from build123d import *

# Parameters (mm, degrees)
SKETCH1_R           = 78.35
SKETCH1_R_2         = 4
SKETCH1_R_3         = 3
SKETCH1_R_4         = 2.5
SKETCH1_W           = 100
SKETCH1_H           = 100
BOSS_EXTRUDE1_DEPTH = 3


with BuildPart() as part:
    # Sketch1 → Boss-Extrude1 (new body)
    with BuildSketch(Plane(origin=(0, 0, 0), x_dir=(1, 0, 0), z_dir=(0, 1, 0))):
        with Locations(Location((0, 0, 0), (0, 0, 270))):
            Circle(SKETCH1_R)
        with Locations(Location((-62.5, 0, 0), (0, 0, 270))):
            Circle(SKETCH1_R_2, mode=Mode.SUBTRACT)
        with Locations(Location((0, -62.5, 0), (0, 0, 270))):
            Circle(SKETCH1_R_3, mode=Mode.SUBTRACT)
        with Locations(Location((0, 62.5, 0), (0, 0, 270))):
            Circle(SKETCH1_R_4, mode=Mode.SUBTRACT)
        with Locations(Location((62.5, 0, 0), (0, 0, 270))):
            Circle(SKETCH1_R_2, mode=Mode.SUBTRACT)
        Rectangle(SKETCH1_W, SKETCH1_H, mode=Mode.SUBTRACT)
    extrude(amount=BOSS_EXTRUDE1_DEPTH)


solid = part.part
Check sheet for the modelled part. Datum: model origin and axes. Units: mm. Give positions to 0.01 mm unless a question says otherwise; leave off trailing zeros. Loops run counter-clockwise (first coordinate to the right, second up) from the corner with the lowest first, then second, coordinate; pieces in that order, holes last. Notation, with made-up numbers: M -10,50.5 L 11,50.5 A27 ccw 11,70.5 Z; hole C 9,-34.5 d9. An arc over 180 degrees is marked long. Use a Markdown table: item, result. Add a question column.
Q1. Sectioned sample at A-A, the plane z = 0. Record the cut outline in (x, y), then the cut area to 3 significant figures.
Q2. Sectioned sample at B-B, the plane x = 0. Record the cut outline in (y, z), then the cut area to 3 significant figures.
Q3. Go/stop test with flat-tipped pins: pin 1 (0.9 mm diameter, centred on y = 2, z = 16.5, fed in from +X); pin 2 (1.5 mm diameter, centred on x = -11.5, y = 1.5, fed in from -Z); pin 3 (4 mm diameter, centred on x = 0, z = -62.5, fed in from +Y); pin 4 (1 mm diameter, centred on x = -57, y = 0.5, fed in from +Z). Record where each tip stops, or that it passes through.
Q4. Sectioned sample at D-D, the plane y = 0.7. Record the cut outline in (x, z).
Q5. Scan lines: line 1 along X through (y, z) = (2.25, 0); line 2 along Z through (x, y) = (-36, 2.05); line 3 along X through (y, z) = (0.7, -16). Record each from-to range of solid material in increasing order. Write a range as [from, to].
Q6. Sectioned sample at C-C, the plane x = 62.5. Record the cut outline in (y, z).
Q7. Mould release check, pull along Z, two halves, no side actions. Record for faces 1 (the cylindrical face through (23.534, 1.479, 74.732)), 2 (the cylindrical face through (-66.405, 1.479, -0.867)), 3 (the flat face through (-51, 3, -1)): pulls with the +Z half, pulls with the -Z half, needs draft (parallel to the pull), parting line crosses it, or undercut.
Verdict:
| question | item | result |
|---|---|---|
| 1 | outline | M -78.35,0 L -66.5,0 L -66.5,3 L -78.35,3 Z; M -58.5,0 L -50,0 L -50,3 L -58.5,3 Z; M 50,0 L 58.5,0 L 58.5,3 L 50,3 Z; M 66.5,0 L 78.35,0 L 78.35,3 L 66.5,3 Z |
| 1 | area | 122 mm^2 |
| 2 | outline | M 0,-78.35 L 3,-78.35 L 3,-65 L 0,-65 Z; M 0,-60 L 3,-60 L 3,-50 L 0,-50 Z; M 0,50 L 3,50 L 3,59.5 L 0,59.5 Z; M 0,65.5 L 3,65.5 L 3,78.35 L 0,78.35 Z |
| 2 | area | 137 mm^2 |
| 3 | pin 1 | x = 76.69 |
| 3 | pin 2 | z = -77.61 |
| 3 | pin 3 | through |
| 3 | pin 4 | z = 54.28 |
| 4 | outline | C 0,0 d156.7; hole C -62.5,0 d8; hole M -50,-50 L 50,-50 L 50,50 L -50,50 Z; hole C 0,62.5 d6; hole C 0,-62.5 d5; hole C 62.5,0 d8 |
| 5 | line 1 | [-78.35, -66.5], [-58.5, -50], [50, 58.5], [66.5, 78.35] |
| 5 | line 2 | [-69.59, -50], [50, 69.59] |
| 5 | line 3 | [-76.7, -50], [50, 76.7] |
| 6 | outline | M 0,-47.25 L 3,-47.25 L 3,-4 L 0,-4 Z; M 0,4 L 3,4 L 3,47.25 L 0,47.25 Z |
| 7 | face 1 | parting line crosses it |
| 7 | face 2 | undercut |
| 7 | face 3 | needs draft |
